Geometry: final body of the model. Coordinates: model frame, mm. A direction names the side the tool comes from. Round coordinates to 2 decimals unless told otherwise and drop trailing zeros. Loops run counter-clockwise (first coordinate to the right, second up) from the corner with the lowest first, then second, coordinate; pieces in that order, holes last. Notation, with made-up numbers: M 42,-25.75 L 78,-25.75 A23 cw 78,-6.75 Z; hole C 27,-29 d2. An arc over 180 degrees is marked long. Return JSON: item names as keys, results as strings.
from build123d import *

# Parameters (mm, degrees)
SKETCH_1_W                  = 11.5
SKETCH_1_H                  = 4
EXTRUDE_1_DEPTH             = 1
SKETCH_2_R                  = 2.9
EXTRUDE_2_DEPTH             = 4
SKETCH_4_R                  = 2.5
EXTRUDE_3_DEPTH             = 3.6
EXTRUDE_4_REACH             = 11.962
SKETCH_5_W                  = 1.8
SKETCH_5_H                  = 6.6
EXTRUDE_4_DIRECTION_2_REACH = 11.962
CUT_EXTRUDE_1_DEPTH         = 10.961551084
CUT_EXTRUDE_1_DEPTH_BACK    = 10.961551084
SKETCH_6_R                  = 1.5
CUT_EXTRUDE_2_DEPTH         = 10.961551084
CUT_EXTRUDE_2_DEPTH_BACK    = 10.961551084
SKETCH_7_W                  = 7.8
SKETCH_7_H                  = 0.6
CHAMFER_1_SIZE              = 1


with BuildPart() as part:
    # 草图1 → 凸台-拉伸1 (new body)
    with BuildSketch(Plane(origin=(0, 0, 0), x_dir=(1, 0, 0), z_dir=(0, 1, 0))):
        Rectangle(SKETCH_1_W, SKETCH_1_H)
    extrude(amount=-EXTRUDE_1_DEPTH)

    # 草图2 → 凸台-拉伸2 (add)
    with BuildSketch(Plane(origin=(0, 0, 0), x_dir=(-1, 0, 0), z_dir=(0, 1, 0))):
        with Locations(Location((0, 0, 0), (0, 0, 90))):
            Circle(SKETCH_2_R)
    extrude(amount=-EXTRUDE_2_DEPTH)

    # 草图3 → 旋转1 (revolve)
    with BuildSketch(Plane.XY, mode=Mode.PRIVATE) as revolve_1_sk:
        with BuildLine():
            Line((0, 0), (2.4, 0))
            Line((2.4, 0), (2.4, 5))
            ThreePointArc((2.4, 5), (1.697056275, 6.697056275), (0, 7.4))
            Line((0, 7.4), (0, 0))
        make_face()
    revolve(revolve_1_sk.sketch.rotate(Axis((0, 7.945806113, 0), (0, -1, 0)), 90), axis=Axis((0, 7.945806113, 0), (0, -1, 0)))

    # 草图4 → 凸台-拉伸3 (add)
    with BuildSketch(Plane.XZ.offset(4)):
        with Locations(Location((0, 0, 0), (0, 0, 90))):
            Circle(SKETCH_4_R)
    extrude(amount=EXTRUDE_3_DEPTH)

    # 凸台-拉伸4: up to this face of the body (flat: up to its plane)
    extrude_4_end = Plane(part.part.faces().sort_by_distance((3.925, -0.5, -2))[0])
    # 草图5 → 凸台-拉伸4 (add, up to the picked face)
    with BuildSketch(Plane.XY, mode=Mode.PRIVATE) as extrude_4_sk1:
        with Locations((-3, -4.3)):
            Rectangle(SKETCH_5_W, SKETCH_5_H)
    extrude_4_tool1 = split(extrude(extrude_4_sk1.sketch, amount=-EXTRUDE_4_REACH, mode=Mode.PRIVATE), bisect_by=extrude_4_end, keep=Keep.BOTH, mode=Mode.PRIVATE)
    # 草图5 → 凸台-拉伸4 (add, up to the picked face)
    with BuildSketch(Plane.XY, mode=Mode.PRIVATE) as extrude_4_sk2:
        with Locations((3, -4.3)):
            Rectangle(SKETCH_5_W, SKETCH_5_H)
    extrude_4_tool2 = split(extrude(extrude_4_sk2.sketch, amount=-EXTRUDE_4_REACH, mode=Mode.PRIVATE), bisect_by=extrude_4_end, keep=Keep.BOTH, mode=Mode.PRIVATE)
    add(extrude_4_tool1.solids().sort_by(Axis((-3, -4.3, 0), (0, 0, -1)))[0])
    add(extrude_4_tool2.solids().sort_by(Axis((3, -4.3, 0), (0, 0, -1)))[0])

    # 凸台-拉伸4 direction 2: up to this face of the body (flat: up to its plane)
    extrude_4_direction_2_end = Plane(part.part.faces().sort_by_distance((3.925, -0.5, 2))[0])
    # 草图5 → 凸台-拉伸4 direction 2 (add, up to the picked face)
    with BuildSketch(Plane.XY, mode=Mode.PRIVATE) as extrude_4_direction_2_sk1:
        with Locations((-3, -4.3)):
            Rectangle(SKETCH_5_W, SKETCH_5_H)
    extrude_4_direction_2_tool1 = split(extrude(extrude_4_direction_2_sk1.sketch, amount=EXTRUDE_4_DIRECTION_2_REACH, mode=Mode.PRIVATE), bisect_by=extrude_4_direction_2_end, keep=Keep.BOTH, mode=Mode.PRIVATE)
    # 草图5 → 凸台-拉伸4 direction 2 (add, up to the picked face)
    with BuildSketch(Plane.XY, mode=Mode.PRIVATE) as extrude_4_direction_2_sk2:
        with Locations((3, -4.3)):
            Rectangle(SKETCH_5_W, SKETCH_5_H)
    extrude_4_direction_2_tool2 = split(extrude(extrude_4_direction_2_sk2.sketch, amount=EXTRUDE_4_DIRECTION_2_REACH, mode=Mode.PRIVATE), bisect_by=extrude_4_direction_2_end, keep=Keep.BOTH, mode=Mode.PRIVATE)
    add(extrude_4_direction_2_tool1.solids().sort_by(Axis((-3, -4.3, 0), (0, 0, 1)))[0])
    add(extrude_4_direction_2_tool2.solids().sort_by(Axis((3, -4.3, 0), (0, 0, 1)))[0])

    # 草图6 → 切除-拉伸1 (cut, two sides: drawn at the far end of the back side and taken through both)
    with BuildSketch(Plane.XY.offset(-CUT_EXTRUDE_1_DEPTH_BACK)):
        with Locations((-5, -3.75)):
            Circle(SKETCH_6_R)
        with Locations((5, -3.75)):
            Circle(SKETCH_6_R)
    extrude(amount=CUT_EXTRUDE_1_DEPTH + CUT_EXTRUDE_1_DEPTH_BACK, mode=Mode.SUBTRACT)

    # 草图7 → 切除-拉伸2 (cut, two sides: drawn at the far end of the back side and taken through both)
    with BuildSketch(Plane.XY.offset(-CUT_EXTRUDE_2_DEPTH_BACK)):
        with Locations((0, -7.3)):
            Rectangle(SKETCH_7_W, SKETCH_7_H)
    extrude(amount=CUT_EXTRUDE_2_DEPTH + CUT_EXTRUDE_2_DEPTH_BACK, mode=Mode.SUBTRACT)

    # 倒角1
    chamfer_1_edges = [part.edges().sort_by_distance(p)[0] for p in [
        (-3.9, -7, 0),
        (3.9, -7, 0),
    ]]
    chamfer(chamfer_1_edges, length=CHAMFER_1_SIZE)


solid = part.part
Q1. Reachability of faces 4 (the flat face through (-3, -3, 2)), 5 (the flat face through (5, -1, 0)), 6 (the flat face through (-5, -1, 0)), 7 (the flat face through (3, -3, -2)), 8 (the flat face through (-3, -3, -2)) from +Z, -Z, +X, -X, +Y, -Y: full face, straight path, thin tool, end or side. Return the list, or none.
Determined:
{"face 4": "+Z, -X, +Y, -Y", "face 5": "+Z, -Z, +X, -Y", "face 6": "+Z, -Z, -X, -Y", "face 7": "-Z, +X, +Y, -Y", "face 8": "-Z, -X, +Y, -Y"}
Q2. Section query D-D (y = 2.75). Output: boundary loops of the cut face in (x, z).
Determined:
{"outline": "C 0,0 d4.8"}
Q3. Section query B-B (x = 0). Output: boundary loops of the cut face in (y, z), plus the area to 3 significant figures.
Determined:
{"outline": "M -7,-2.5 L -4,-2.5 L -4,-2.9 L 0,-2.9 L 0,-2.4 L 5,-2.4 A2.4 ccw 5,2.4 L 0,2.4 L 0,2.9 L -4,2.9 L -4,2.5 L -7,2.5 Z", "area": "71.2 mm^2"}
Q4. Pin query (flat end, axial travel): pin 1 (1.4 mm diameter, centred on y = -5, z = 0, fed in from -X); pin 2 (0.6 mm diameter, centred on y = -5, z = 0.5, fed in from +X); pin 3 (1.5 mm diameter, centred on x = 2, y = -1, fed in from -Z). Return the tip coordinate at first contact, or that it passes through.
Determined:
{"pin 1": "stops at x = -3.9", "pin 2": "stops at x = 3.9", "pin 3": "stops at z = -2.62"}
Q5. Section query C-C (y = -0.5). Output: boundary loops of the cut face in (x, z).
Determined:
{"outline": "M -5.75,-2 L -2.1,-2 A2.9 ccw 2.1,-2 L 5.75,-2 L 5.75,2 L 2.1,2 A2.9 ccw -2.1,2 L -5.75,2 Z"}
Q6. Section query A-A (z = 0). Output: boundary loops of the cut face in (x, y), plus the area to 3 significant figures.
Determined:
{"outline": "M -5.75,-1 L -3.9,-1 L -3.9,-2.73 A1.5 cw -3.9,-4.77 L -3.9,-6 L -2.9,-7 L 2.9,-7 L 3.9,-6 L 3.9,-4.77 A1.5 cw 3.9,-2.73 L 3.9,-1 L 5.75,-1 L 5.75,0 L 2.4,0 L 2.4,5 A2.4 ccw -2.4,5 L -2.4,0 L -5.75,0 Z", "area": "89.2 mm^2"}
Q7. Pull-direction query (X, two-part tool) for faces 1 (the flat face through (-0.1, -4, 2.7)), 2 (the cylindrical face through (-2.024, 2.535, 1.29)), 3 (the cylindrical face through (3.5, -3.7, 0)); classes: pulls with the +X half, pulls with the -X half, needs draft (parallel to the pull), parting line crosses it, or undercut.
Determined:
{"face 1": "undercut", "face 2": "parting line crosses it", "face 3": "pulls with the +X half"}
Q8. Material intervals for L1, parallel to X at y = -2, z = 1.5; L2, parallel to Y at x = 5.25, z = -1.45; L3, parallel to Z at x = 2.5, y = -4.25, sorted ascending.
Determined:
{"L1": "x = -3.9 to 3.9", "L2": "y = -1 to 0", "L3": "z = -2 to 2"}
